```python
from build123d import *

# Parameters (mm, degrees)
F1_DEPTH = 80
F2_DEPTH = 8
F4_DEPTH = 3
F7_DEPTH = 80.001
F8_DEPTH = 80.001


with BuildPart() as f1:
    # F0 (on Top) → F1 (new body)
    with BuildSketch(Plane.XY):
        with BuildLine():
            Line((35, 40), (-35, 40))
            ThreePointArc((-35, 40), (-38.535534, 38.535534), (-40, 35))
            Line((-40, 35), (-40, -35))
            ThreePointArc((-40, -35), (-38.535534, -38.535534), (-35, -40))
            Line((-35, -40), (35, -40))
            ThreePointArc((35, -40), (38.535534, -38.535534), (40, -35))
            Line((40, -35), (40, 35))
            ThreePointArc((40, 35), (38.535534, 38.535534), (35, 40))
        make_face()
        with BuildLine():
            ThreePointArc((-36, 31), (-34.535534, 34.535534), (-31, 36))
            Line((-31, 36), (31, 36))
            ThreePointArc((31, 36), (34.535534, 34.535534), (36, 31))
            Line((36, 31), (36, -31))
            ThreePointArc((36, -31), (34.535534, -34.535534), (31, -36))
            Line((31, -36), (-31, -36))
            ThreePointArc((-31, -36), (-34.535534, -34.535534), (-36, -31))
            Line((-36, -31), (-36, 31))
        make_face(mode=Mode.SUBTRACT)
    extrude(amount=F1_DEPTH)

    # F0 (on Top) → F2 (join)
    with BuildSketch(Plane.XY):
        with BuildLine():
            Line((31, 36), (-31, 36))
            ThreePointArc((-31, 36), (-34.535534, 34.535534), (-36, 31))
            Line((-36, 31), (-36, -31))
            ThreePointArc((-36, -31), (-34.535534, -34.535534), (-31, -36))
            Line((-31, -36), (31, -36))
            ThreePointArc((31, -36), (34.535534, -34.535534), (36, -31))
            Line((36, -31), (36, 31))
            ThreePointArc((36, 31), (34.535534, 34.535534), (31, 36))
        make_face()
    extrude(amount=F2_DEPTH)

    # F3 (on face) → F4 (join)
    with BuildSketch(Plane.XY.offset(80)):
        with BuildLine():
            Line((33, 38), (-33, 38))
            ThreePointArc((-33, 38), (-36.535534, 36.535534), (-38, 33))
            Line((-38, 33), (-38, -33))
            ThreePointArc((-38, -33), (-36.535534, -36.535534), (-33, -38))
            Line((-33, -38), (33, -38))
            ThreePointArc((33, -38), (36.535534, -36.535534), (38, -33))
            Line((38, -33), (38, 33))
            ThreePointArc((38, 33), (36.535534, 36.535534), (33, 38))
        make_face()
        with BuildLine():
            Line((-36, -31), (-36, 31))
            ThreePointArc((-36, 31), (-34.535534, 34.535534), (-31, 36))
            Line((-31, 36), (31, 36))
            ThreePointArc((31, 36), (34.535534, 34.535534), (36, 31))
            Line((36, 31), (36, -31))
            ThreePointArc((36, -31), (34.535534, -34.535534), (31, -36))
            Line((31, -36), (-31, -36))
            ThreePointArc((-31, -36), (-34.535534, -34.535534), (-36, -31))
        make_face(mode=Mode.SUBTRACT)
    extrude(amount=F4_DEPTH)

    # F6 (on face) → F7 (cut, through all)
    with BuildSketch(Plane(origin=(0, 40, 0), x_dir=(-1, 0, 0), z_dir=(0, 1, 0))):
        with BuildLine():
            Line((-25, 56), (-10, 56))
            ThreePointArc((-10, 56), (-6.464466, 57.464466), (-5, 61))
            Line((-5, 61), (-5, 71))
            ThreePointArc((-5, 71), (-6.464466, 74.535534), (-10, 76))
            Line((-10, 76), (-25, 76))
            ThreePointArc((-25, 76), (-28.535534, 74.535534), (-30, 71))
            Line((-30, 71), (-30, 61))
            ThreePointArc((-30, 61), (-28.535534, 57.464466), (-25, 56))
        make_face()
        with BuildLine():
            ThreePointArc((5, 61), (6.464466, 57.464466), (10, 56))
            Line((10, 56), (25, 56))
            ThreePointArc((25, 56), (28.535534, 57.464466), (30, 61))
            Line((30, 61), (30, 71))
            ThreePointArc((30, 71), (28.535534, 74.535534), (25, 76))
            Line((25, 76), (10, 76))
            ThreePointArc((10, 76), (6.464466, 74.535534), (5, 71))
            Line((5, 71), (5, 61))
        make_face()
    extrude(amount=-F7_DEPTH, mode=Mode.SUBTRACT)

    # F5 (on face) → F8 (cut, through all)
    with BuildSketch(Plane.YZ.offset(40)):
        with BuildLine():
            Line((-25, 56), (-10, 56))
            ThreePointArc((-10, 56), (-6.464466, 57.464466), (-5, 61))
            Line((-5, 61), (-5, 71))
            ThreePointArc((-5, 71), (-6.464466, 74.535534), (-10, 76))
            Line((-10, 76), (-25, 76))
            ThreePointArc((-25, 76), (-28.535534, 74.535534), (-30, 71))
            Line((-30, 71), (-30, 61))
            ThreePointArc((-30, 61), (-28.535534, 57.464466), (-25, 56))
        make_face()
        with BuildLine():
            ThreePointArc((5, 61), (6.464466, 57.464466), (10, 56))
            Line((10, 56), (25, 56))
            ThreePointArc((25, 56), (28.535534, 57.464466), (30, 61))
            Line((30, 61), (30, 71))
            ThreePointArc((30, 71), (28.535534, 74.535534), (25, 76))
            Line((25, 76), (10, 76))
            ThreePointArc((10, 76), (6.464466, 74.535534), (5, 71))
            Line((5, 71), (5, 61))
        make_face()
    extrude(amount=-F8_DEPTH, mode=Mode.SUBTRACT)


solid = f1.part
```
Input: part model. Units: mm. Frame: model coordinates. A direction names the side the tool comes from. Give positions to 0.01 mm unless a question says otherwise; leave off trailing zeros. Loops run counter-clockwise (first coordinate to the right, second up) from the corner with the lowest first, then second, coordinate; pieces in that order, holes last. Notation, with made-up numbers: (41.5, 47) -> (92.5, 47) arc R9 ccw to (92.5, 64) -> close; hole circle Ø10 at (32.25, 76). An arc over 180 degrees is marked (long way). Use a Markdown table: item, result.
Q1. Ray query, probe 1 along Y at (x, z) = (15, 13.5); probe 2 along Z at (x, y) = (17, -21.5). Return the intervals inside material, ascending. Write a range as from..to.
Entries:
| item | result |
|---|---|
| probe 1 | y = -40..-36, 36..40 |
| probe 2 | z = 0..8 |
Q2. Pull-direction query (X, two-part tool) for faces 5 (the cylindrical face through (37, 36, 81)), 6 (the flat face through (38, 17, 56)), 7 (the flat face through (-18, 38, 76)), 8 (the flat face through (-36, 0, 37)); classes: pulls with the +X half, pulls with the -X half, needs draft (parallel to the pull), parting line crosses it, or undercut.
Entries:
| item | result |
|---|---|
| face 5 | pulls with the +X half |
| face 6 | needs draft |
| face 7 | undercut |
| face 8 | undercut |
Q3. Section query B-B, the plane z = 27. Return the cut outline in (x, y).
Entries:
| item | result |
|---|---|
| outline | (-40, -35) arc R5 ccw to (-35, -40) -> (35, -40) arc R5 ccw to (40, -35) -> (40, 35) arc R5 ccw to (35, 40) -> (-35, 40) arc R5 ccw to (-40, 35) -> close; hole (-36, -31) arc R5 ccw to (-31, -36) -> (31, -36) arc R5 ccw to (36, -31) -> (36, 31) arc R5 ccw to (31, 36) -> (-31, 36) arc R5 ccw to (-36, 31) -> close |
Q4. Section query D-D, the plane y = 3. Return the cut outline in (x, z).
Entries:
| item | result |
|---|---|
| outline | (-40, 0) -> (40, 0) -> (40, 80) -> (38, 80) -> (38, 83) -> (36, 83) -> (36, 8) -> (-36, 8) -> (-36, 83) -> (-38, 83) -> (-38, 80) -> (-40, 80) -> close |
Q5. Access query for faces 1 (the flat face through (-5, -38, 66)), 2 (the cylindrical face through (39, 38, 39)), 3 (the cylindrical face through (38, -6, 74)), 4 (the flat face through (-0.2, -38.3, 80)). Directions: +Z, -Z, +X, -X, +Y, -Y. A direction counts if a zero-diameter tool reaches every point of the face in a straight line with its end or side. Return the directions, or none.
Entries:
| item | result |
|---|---|
| face 1 | +Y, -Y |
| face 2 | +Z, -Z, +X, +Y |
| face 3 | +X, -X |
| face 4 | +Z |
Q6. First-contact query: P1, Ø3, axis at x = -13, y = -30.5, coming from the +Z side; P2, Ø4.5, axis at y = 38, z = 67.5, coming from the -X side; P3, Ø3, axis at x = -38.5, z = 65.5, coming from the +Y side; P4, Ø1.2, axis at x = -17, y = -38, coming from the -Z side. Flat tips, straight axial feed; report the tip coordinate or a pass-through.
Entries:
| item | result |
|---|---|
| P1 | stops at z = 8 |
| P2 | stops at x = -39.94 |
| P3 | stops at y = 39.58 |
| P4 | stops at z = 0 |
Q7. Section query A-A, the plane x = 18. Return the cut outline in (y, z), plus the area to 3 significant figures.
Entries:
| item | result |
|---|---|
| outline | (-40, 0) -> (40, 0) -> (40, 56) -> (36, 56) -> (36, 8) -> (-36, 8) -> (-36, 56) -> (-40, 56) -> close; (-40, 76) -> (-36, 76) -> (-36, 83) -> (-38, 83) -> (-38, 80) -> (-40, 80) -> close; (36, 76) -> (40, 76) -> (40, 80) -> (38, 80) -> (38, 83) -> (36, 83) -> close |
| area | 1,070 mm² |
